Here's the drawing with two shaded views (mm, measured from the low corner). I have some questions. Coordinates: 2 decimals unless noted, no trailing zeros. Write each loop counter-clockwise with the first axis right and the second up, starting at its lowest first coordinate (ties: lowest second). Pieces come first, ordered by that corner, then holes.
Item 1: If we section it at A-A (y = 12.7): Please give me the cut outline in (x, z) (3 decimals).
Item 2: We'd pull the mould along X, two halves only. Please class the marked faces 1 and 2: +X half, -X half, draft (parallel to the pull), parting line (faces both ways), or undercut.
Item 3: If I drill on line 1 (Y direction, x = 147.32, z = 4.5); line 2 (X direction, y = 17.5, z = 4.75), over which ranges is the centre line in solid material (lowest first)?
Item 4: If we section it at B-B (x = 12.7): Please give me the cut outline in (y, z) (3 decimals).
Item 5: If we section it at C-C (z = 7): Please give me the cut outline in (x, y), then the cut area to 3 significant figures.
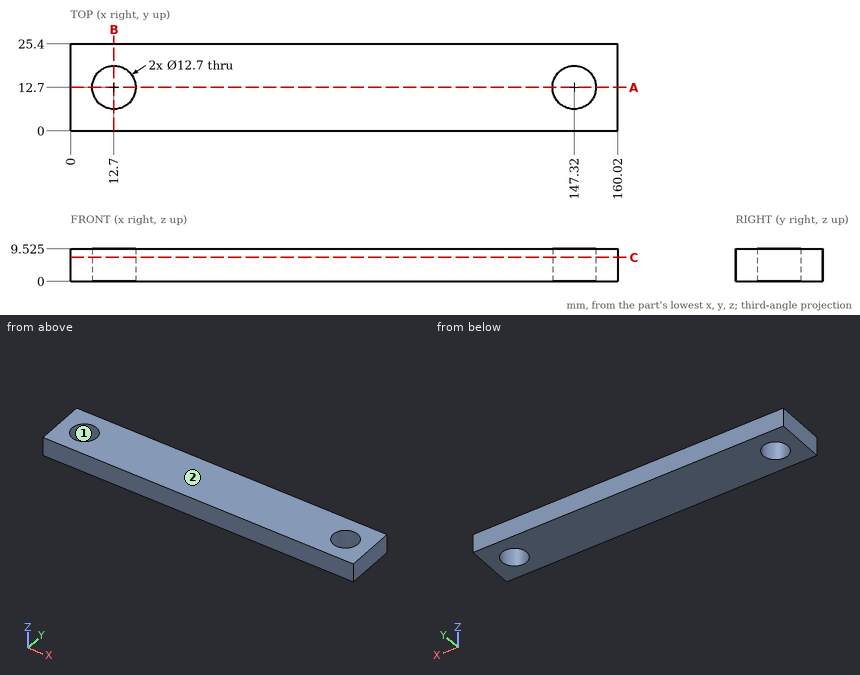
Answer list:
1. outline: (0, 0) - (6.35, 0) - (6.35, 9.525) - (0, 9.525) - close; (19.05, 0) - (140.97, 0) - (140.97, 9.525) - (19.05, 9.525) - close; (153.67, 0) - (160.02, 0) - (160.02, 9.525) - (153.67, 9.525) - close
2. face 1: undercut
2. face 2: draft
3. line 1: y = 0 to 6.35, 19.05 to 25.4
3. line 2: x = 0 to 8.54, 16.86 to 143.16, 151.48 to 160.02
4. outline: (0, 0) - (6.35, 0) - (6.35, 9.525) - (0, 9.525) - close; (19.05, 0) - (25.4, 0) - (25.4, 9.525) - (19.05, 9.525) - close
5. outline: (0, 0) - (160.02, 0) - (160.02, 25.4) - (0, 25.4) - close; hole circle Ø12.7 at (12.7, 12.7); hole circle Ø12.7 at (147.32, 12.7)
5. area: 3,810 mm2
